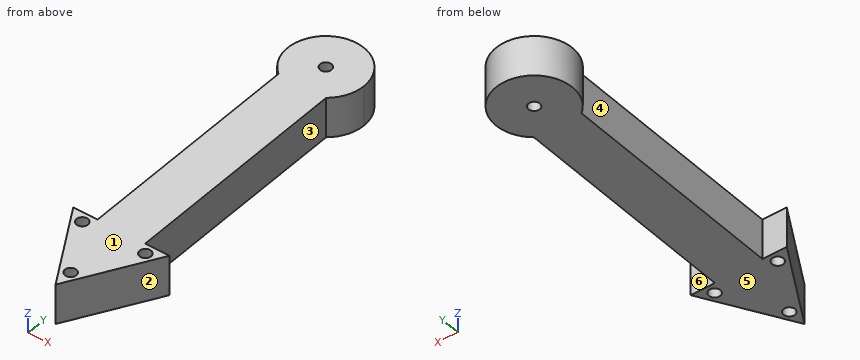
```python
from build123d import *

# Parameters (mm, degrees)
F0_R     = 1.5
F1_DEPTH = 10.5


with BuildPart() as f1:
    # F0 (on Top) → F1 (new body)
    with BuildSketch(Plane.XY):
        with BuildLine():
            ThreePointArc((6.249218, 30.291278), (9.013661, 33.767573), (10, 38.098151))
            ThreePointArc((10, 38.098151), (-4.330578, 47.111813), (-6.249218, 30.291278))
            ThreePointArc((-6.249218, 30.291278), (0, 28.098151), (6.249218, 30.291278))
        make_face()
        with Locations((0, 38.098151)):
            Circle(F0_R, mode=Mode.SUBTRACT)
        with BuildLine():
            ThreePointArc((6.249218, 30.291278), (0, 28.098151), (-6.249218, 30.291278))
            Line((-6.249218, 30.291278), (-6.249218, -29.708722))
            Line((-6.249218, -29.708722), (6.249218, -29.708722))
            Line((6.249218, -29.708722), (6.249218, 30.291278))
        make_face()
        Polygon((6.249218, -29.708722), (-6.249218, -29.708722), (-12.60285, -29.708722), (0, -51.537499), (12.60285, -29.708722), align=None)
        with Locations((-8.272723, -32.208722)):
            Circle(F0_R, mode=Mode.SUBTRACT)
        with Locations((0, -46.537499)):
            Circle(F0_R, mode=Mode.SUBTRACT)
        with Locations((8.272723, -32.208722)):
            Circle(F0_R, mode=Mode.SUBTRACT)
    extrude(amount=F1_DEPTH)


solid = f1.part
```
Build history of the part. All positions in model axes, mm. Face numbers are marked on the shaded views. A direction names the side the tool comes from. Give positions to 0.01 mm unless a question says otherwise; leave off trailing zeros. Loops run counter-clockwise (first coordinate to the right, second up) from the corner with the lowest first, then second, coordinate; pieces in that order, holes last. Notation, with made-up numbers: (83, 41) - (92, 41) arc R31 ccw to (92, 67) - close; hole circle Ø10 at (5.5, 71.5). An arc over 180 degrees is marked (long way). Use a Markdown table: item, result.
(1) Which spindle directions (+Z, -Z, +X, -X, +Y, -Y) get a long thin tool onto all of the face, cutting with end or side? Do the marked faces 4, 5 and 6. Say none if no direction does.
Taken from the geometry:
| item | result |
|---|---|
| face 4 | +Z, -Z, -X |
| face 5 | -Z, +X, -X, +Y, -Y |
| face 6 | +Z, -Z, +X |
(2) Wall check: line 1 along X through (y, z) = (-32, 7); line 2 along X through (y, z) = (-33, 5.75); line 3 along Y through (x, z) = (-7.5, 3.5). Give the ranges that are in metal, low to high.
Taken from the geometry:
| item | result |
|---|---|
| line 1 | -11.28 to -9.76, -6.79 to 6.79, 9.76 to 11.28 |
| line 2 | -10.7 to -9.55, -7 to 7, 9.55 to 10.7 |
| line 3 | -38.55 to -33.49, -30.92 to -29.71, 31.48 to 44.71 |
(3) Band-saw the part on C-C (y = -3). Give the cut face in (x, z), and give its area (3 significant figures).
Taken from the geometry:
| item | result |
|---|---|
| outline | (-6.25, 0) - (6.25, 0) - (6.25, 10.5) - (-6.25, 10.5) - close |
| area | 131 mm2 |
(4) Band-saw the part on A-A (x = 7.75). Give the cut face in (y, z).
Taken from the geometry:
| item | result |
|---|---|
| outline | (-38.11, 0) - (-33.61, 0) - (-33.61, 10.5) - (-38.11, 10.5) - close; (-30.8, 0) - (-29.71, 0) - (-29.71, 10.5) - (-30.8, 10.5) - close; (31.78, 0) - (44.42, 0) - (44.42, 10.5) - (31.78, 10.5) - close |
(5) Band-saw the part on D-D (x = -3.25). Give the cut face in (y, z).
Taken from the geometry:
| item | result |
|---|---|
| outline | (-45.91, 0) - (47.56, 0) - (47.56, 10.5) - (-45.91, 10.5) - close |
(6) Pull direction Y, two halves, no side cores. Call the marked faces 1, 2 and 3: +Y half, -Y half, draft (parallel to the pull), parting line (faces both ways), or undercut.
Taken from the geometry:
| item | result |
|---|---|
| face 1 | draft |
| face 2 | -Y half |
| face 3 | undercut |
(7) Drop flat-ended pins along their axis: pin 1 Ø1 at (y, z) = (5.5, 6.5) entering from -X; pin 2 Ø2 at (x, z) = (-3.5, 6.5) entering from -Y; pin 3 Ø1 at (x, z) = (-1, 5.5) entering from -Y. Give the stop position or say it passes through.
Taken from the geometry:
| item | result |
|---|---|
| pin 1 | x = -6.25 |
| pin 2 | y = -47.21 |
| pin 3 | y = -50.67 |
(8) Band-saw the part on B-B (z = 1.5). Give the cut face in (x, y).
Taken from the geometry:
| item | result |
|---|---|
| outline | (-12.6, -29.71) - (0, -51.54) - (12.6, -29.71) - (6.25, -29.71) - (6.25, 30.29) arc R10 ccw to (10, 38.1) arc R10 ccw (long way) to (-6.25, 30.29) - (-6.25, -29.71) - close; hole circle Ø3 at (-8.27, -32.21); hole circle Ø3 at (0, -46.54); hole circle Ø3 at (0, 38.1); hole circle Ø3 at (8.27, -32.21) |
